Check sheet for the modelled part. Datum: model origin and axes. Units: mm. A direction names the side the tool comes from. Give positions to 0.01 mm unless a question says otherwise; leave off trailing zeros. Loops run counter-clockwise (first coordinate to the right, second up) from the corner with the lowest first, then second, coordinate; pieces in that order, holes last. Notation, with made-up numbers: M -39,70 L -8,70 A22 cw -8,107 Z; hole C -19,11 d2. An arc over 180 degrees is marked long. One line per question, with ' | ' between items. Start each with the question number.
from build123d import *

# Parameters (mm, degrees)
F0_W     = 15
F0_H     = 15
F1_DEPTH = 20
F2_DEPTH = 40
F4_DEPTH = 20
F6_DEPTH = 20


with BuildPart() as f1:
    # F0 (on Right) → F1 (new body)
    with BuildSketch(Plane.YZ):
        with Locations((7.5, 7.5)):
            Rectangle(F0_W, F0_H)
        with Locations((22.5, 7.5)):
            Rectangle(F0_W, F0_H)
        with Locations((7.5, 22.5)):
            Rectangle(F0_W, F0_H)
        with Locations((22.5, 22.5)):
            Rectangle(F0_W, F0_H)
    extrude(amount=F1_DEPTH)

    # F0 (on Right) → F2 (join)
    with BuildSketch(Plane.YZ):
        with Locations((22.5, 7.5)):
            Rectangle(F0_W, F0_H)
        with Locations((22.5, 22.5)):
            Rectangle(F0_W, F0_H)
        with Locations((7.5, 22.5)):
            Rectangle(F0_W, F0_H)
    extrude(amount=F2_DEPTH)

    # F3 (on face) → F4 (cut)
    with BuildSketch(Plane.YZ.offset(40)):
        Polygon((30, 30), (15, 30), (30, 0), align=None)
    extrude(amount=-F4_DEPTH, mode=Mode.SUBTRACT)

    # F5 (on face) → F6 (join)
    with BuildSketch(Plane.YZ.offset(20)):
        Polygon((15, 15), (0, 15), (15, 0), align=None)
    extrude(amount=F6_DEPTH)


solid = f1.part
Q1. Cross-section at C-C (x = 27). Record the cut outline in (y, z), and give its area (4 significant figures).
Q2. Depth check by flat-ended pin: P1, Ø3, axis at y = 19.5, z = 27, coming from the +X side. Enter the tip coordinate at first touch or a pass-through.
Q3. Cross-section at B-B (y = 26.5). Record the cut outline in (x, z).
Q4. Access from +Z, -Z, +X, -X, +Y, -Y to the whole of each face (thin tool, end or side, straight path). Record for faces 1 (the flat face through (0, 15, 15)), 2 (the flat face through (20, 26, 22)), 3 (the flat face through (20, 4, 4)).
Q5. Material ranges on probe 1 along X at (y, z) = (28, 11.25); probe 2 along Y at (x, z) = (21, 24.5), recorded low to high. Write a range as from..to.
Q6. Cross-section at D-D (z = 8.5). Record the cut outline in (x, y), and give its area (3 significant figures).
Q7. Cross-section at A-A (z = 12.5). Record the cut outline in (x, y), and give its area (4 significant figures).
Solved:
1) outline: M 0,15 L 15,0 L 30,0 L 15,30 L 0,30 Z | area: 562.5 mm²
2) P1: stops at x = 20
3) outline: M 0,0 L 40,0 L 40,7 L 20,7 L 20,30 L 0,30 Z
4) face 1: +Z, -Z, -X, +Y, -Y | face 2: +Z, +X, +Y | face 3: -Z, +X, -Y
5) probe 1: x = 0..20 | probe 2: y = 0..17.75
6) outline: M 0,0 L 20,0 L 20,6.5 L 40,6.5 L 40,25.75 L 20,25.75 L 20,30 L 0,30 Z | area: 985 mm²
7) outline: M 0,0 L 20,0 L 20,2.5 L 40,2.5 L 40,23.75 L 20,23.75 L 20,30 L 0,30 Z | area: 1,025 mm²
